Part print with two shaded views. Sizes in mm from the minimum x, y, z corner. A direction names the side the tool comes from. Round coordinates to 2 decimals unless told otherwise and drop trailing zeros. Loops run counter-clockwise (first coordinate to the right, second up) from the corner with the lowest first, then second, coordinate; pieces in that order, holes last.
(1) Cut at B-B on z = 5. List the corners of the cut face in (x, y) (1 decimal).
(2) Probe probe 1 along Y at (x, z) = (6.25, 7.75); probe 2 along X at (y, z) = (4.25, 5.5) (1 decimal); probe 3 along Z at (x, y) = (5.75, 0.75) (1 decimal). List the from-to ranges inside material, lowest first.
(3) Cut at D-D on y = 4. List the corners of the cut face in (x, z), then the cut area to 3 significant figures.
(4) Tool access for the marked faces 1 and 2: list every direction of +Z, -Z, +X, -X, +Y, -Y with a clear straight run to the whole face (end or side of a thin tool).
(5) Flat gauge pin, fed straight in: pin 1 (1.5 mm diameter, centred on x = 8, z = 7.5, fed in from -Y). Where does the tip first touch, or does it go through?
(6) Cut at C-C on x = 1. List the corners of the cut face in (y, z).
(7) Cut at A-A on y = 5.5. List the corners of the cut face in (x, z).
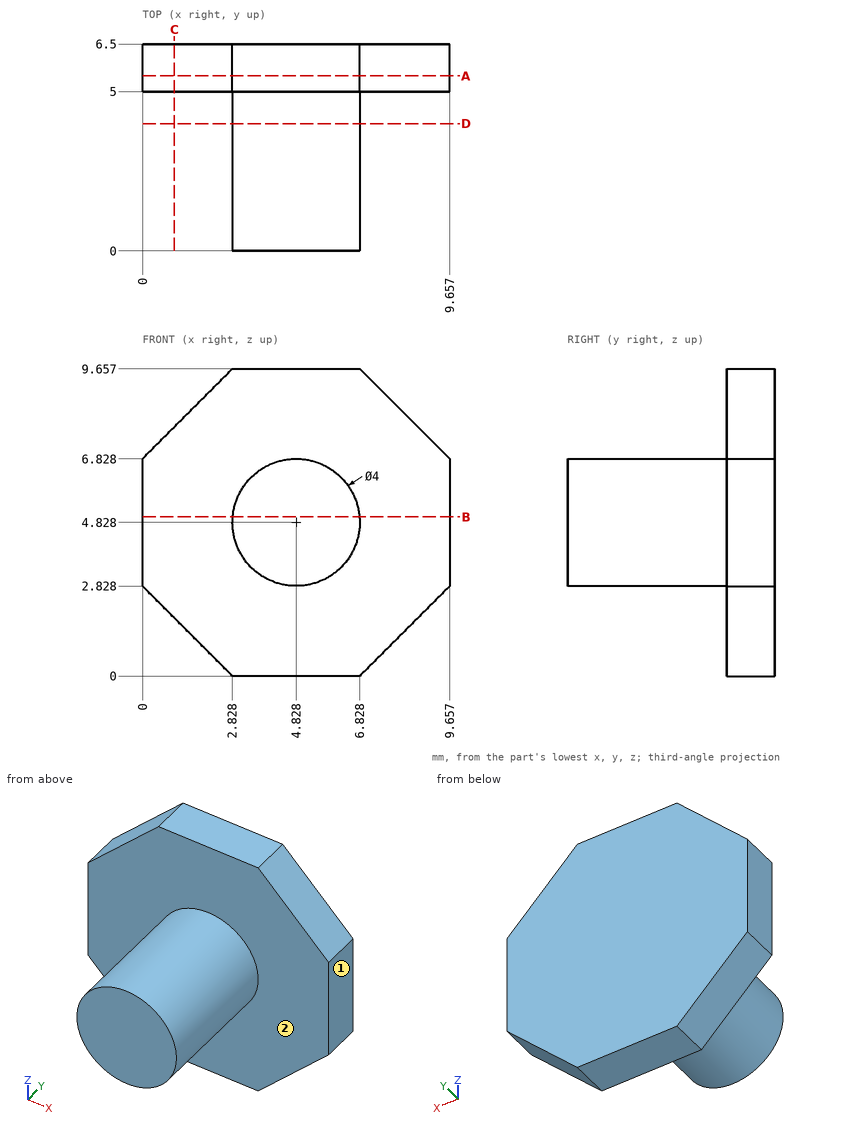
Final values:
1. outline: (0, 5) - (2.8, 5) - (2.8, 0) - (6.8, 0) - (6.8, 5) - (9.7, 5) - (9.7, 6.5) - (0, 6.5) - close
2. probe 1: y = 5 to 6.5
2. probe 2: x = 2.9 to 6.7
2. probe 3: z = 3.1 to 6.6
3. outline: circle Ø4 at (4.83, 4.83)
3. area: 12.6 mm2
4. face 1: +Z, -Z, +X, +Y, -Y
4. face 2: -Y
5. pin 1: stops at y = 5
6. outline: (5, 1.83) - (6.5, 1.83) - (6.5, 7.83) - (5, 7.83) - close
7. outline: (0, 2.83) - (2.83, 0) - (6.83, 0) - (9.66, 2.83) - (9.66, 6.83) - (6.83, 9.66) - (2.83, 9.66) - (0, 6.83) - close
